The listing builds one solid part. Answer for the finished solid, in the listing's coordinates (mm). Face numbers are marked on the shaded views. A direction names the side the tool comes from. Round coordinates to 2 decimals unless told otherwise and drop trailing zeros. Loops run counter-clockwise (first coordinate to the right, second up) from the corner with the lowest first, then second, coordinate; pieces in that order, holes last. Notation, with made-up numbers: M -8.5,-25.5 L 4.5,-25.5 A25 ccw 4.5,9.5 Z; hole C -9.5,-14.75 d10. An arc over 180 degrees is marked long. Put each result on its own line as item: value. Start each with the question number.
(1) Section D-D, the plane x = -91 is taken. Determine the outline of the cut face in (y, z), then the cut area to 3 significant figures.
(2) Section A-A, the plane y = 0 is taken. Determine the outline of the cut face in (x, z).
(3) Determine the mould class of the marked faces 1, 2 and 3 for opening direction Y: released by +Y, released by -Y, zero draft, split by the parting line, or undercut.
(4) Section C-C, the plane x = -66 is taken. Determine the outline of the cut face in (y, z), then the cut area to 3 significant figures.
(5) Straight lines are drawn through the part: line 1 (Y direction, x = -76, z = 2.5); line 2 (Z direction, x = -0.5, y = 21.5). For each, find the intervals that lie inside material, in ascending order.
(6) Which of the six approach directions +Z, -Z, +X, -X, +Y, -Y give full straight-line access (tool end or side, diameter ignored) to the marked faces 4 and 5?
(7) Section B-B, the plane z = 33.5 is taken. Determine the outline of the cut face in (x, y).
(8) Flat-ended cylindrical pins translate along their axes: P1, Ø3.5, axis at x = -7.17, y = -12.7, coming from the +Z side; P2, Ø3, axis at x = -74, z = 16.25, coming from the -Y side; P3, Ø0.8, axis at y = 39.5, z = 18.5, coming from the +X side; P4, Ø1.2, axis at x = -102.5, y = -39.5, coming from the +Z side. Find the tip coordinate at first contact, or state that the pin passes through.
```python
from build123d import *

# Parameters (mm, degrees)
F0_R     = 6.35
F0_R_2   = 1.4732
F1_DEPTH = 1.524
F2_W     = 66.04
F2_H     = 1.524
F3_DEPTH = 38.1
F4_W     = 40.64
F4_H     = 25.4
F4_R     = 1.6383
F5_DEPTH = 1.524


with BuildPart() as f1:
    # F0 (on Top) → F1 (new body)
    with BuildSketch(Plane.XY):
        Polygon((11.91761, 0), (11.91761, 38.1), (-64.28239, 38.732044), (-130.32239, 38.732044), (-130.32239, 0), (-130.32239, -37.783978), (11.91761, -38.1), align=None)
        with Locations((-92.262112, 0)):
            Circle(F0_R, mode=Mode.SUBTRACT)
        with Locations((-20.401943, -12.703063)):
            Circle(F0_R_2, mode=Mode.SUBTRACT)
        with Locations((-7.168442, -12.703063)):
            Circle(F0_R_2, mode=Mode.SUBTRACT)
        with Locations((-20.401943, 12.703063)):
            Circle(F0_R_2, mode=Mode.SUBTRACT)
        with Locations((-7.168442, 12.703063)):
            Circle(F0_R_2, mode=Mode.SUBTRACT)
        Polygon((-64.28239, -38.1), (11.91761, -38.1), (-130.32239, -37.783978), align=None)
    extrude(amount=F1_DEPTH)

    # F2 (on Top) → F3 (join)
    with BuildSketch(Plane.XY):
        with Locations((-97.30239, 39.494044)):
            Rectangle(F2_W, F2_H)
    extrude(amount=F3_DEPTH)

    # F4 (on face) → F5 (cut)
    with BuildSketch(Plane.XZ.offset(-38.732044)):
        with Locations((-97.30239, 25.4)):
            Rectangle(F4_W, F4_H)
        with Locations((-120.988675, 28.948788)):
            Circle(F4_R)
        with Locations((-120.988675, 16.248788)):
            Circle(F4_R)
        with Locations((-73.998675, 16.248788)):
            Circle(F4_R)
        with Locations((-73.998675, 28.948788)):
            Circle(F4_R)
    extrude(amount=-F5_DEPTH, mode=Mode.SUBTRACT)

    # F6: F1 across plane


with BuildPart() as f1_1:
    add(f1.part)
    add(f1.part.mirror(Plane.XZ))


solid = f1_1.part
```
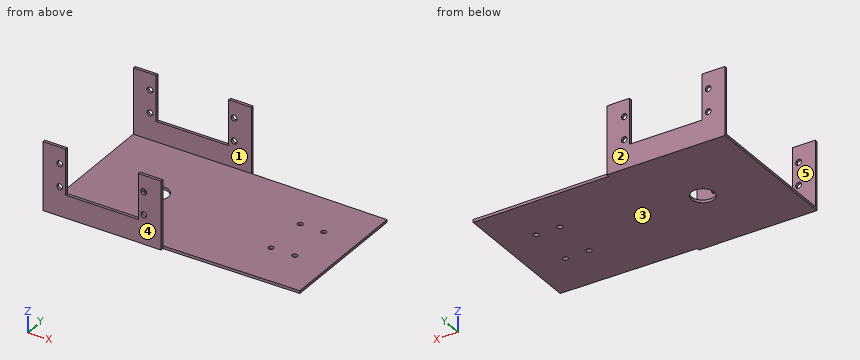
Recorded:
1. outline: M -40.26,0 L -6.22,0 L -6.22,1.52 L -38.73,1.52 L -38.73,12.7 L -40.26,12.7 Z; M 6.22,0 L 40.26,0 L 40.26,12.7 L 38.73,12.7 L 38.73,1.52 L 6.22,1.52 Z
1. area: 138 mm²
2. outline: M -130.32,0 L -98.61,0 L -98.61,1.52 L -130.32,1.52 Z; M -85.91,0 L 11.92,0 L 11.92,1.52 L -85.91,1.52 Z
3. face 1: undercut
3. face 2: released by +Y
3. face 3: zero draft
4. outline: M -40.26,0 L 40.26,0 L 40.26,38.1 L 38.73,38.1 L 38.73,1.52 L -38.73,1.52 L -38.73,38.1 L -40.26,38.1 Z
4. area: 234 mm²
5. line 1: y = -40.26 to -38.73, 38.73 to 40.26
5. line 2: z = 0 to 1.52
6. face 4: +Z, -Z, +X, -X, -Y
6. face 5: +Z, +X, -X
7. outline: M -130.32,-40.26 L -117.62,-40.26 L -117.62,-38.73 L -130.32,-38.73 Z; M -130.32,38.73 L -117.62,38.73 L -117.62,40.26 L -130.32,40.26 Z; M -76.98,-40.26 L -64.28,-40.26 L -64.28,-38.73 L -76.98,-38.73 Z; M -76.98,38.73 L -64.28,38.73 L -64.28,40.26 L -76.98,40.26 Z
8. P1: stops at z = 1.52
8. P2: passes through
8. P3: stops at x = -64.28
8. P4: stops at z = 12.7
